Here's the drawing with two shaded views (mm, measured from the low corner). I have some questions. Round coordinates to 2 decimals unless told otherwise and drop trailing zeros. Write each loop counter-clockwise with the first axis right and the second up, starting at its lowest first coordinate (ties: lowest second). Pieces come first, ordered by that corner, then holes. Notation, with made-up numbers: M 62.25,89.25 L 68.25,89.25 A25 cw 68.25,127.25 Z; hole C 46,-38 d11. An arc over 180 degrees is marked long. Answer as a JSON object with one key per item and string values. Group by question number.
1) Suppose I cut it at B-B, the plane x = 28. Write out the boundary of the cut face in (y, z).
2) Suppose I cut it at C-C, the plane y = 21.5. Write out the boundary of the cut face in (x, z), and give its area (3 significant figures).
3) I'm going to push flat-ended pins straight in: pin 1 Ø1 at (y, z) = (2.5, 2.5) entering from -X; pin 2 Ø0.9 at (x, z) = (26.5, 1) entering from +Y. Where does each tip first touch, or does it pass through?
4) Please list where these lines run through material, in increasing order: L1, parallel to X at y = 23.75, z = 2.3; L2, parallel to X at y = 5, z = 1.1; L3, parallel to Y at x = 27, z = 1.6. Write a range as [from, to].
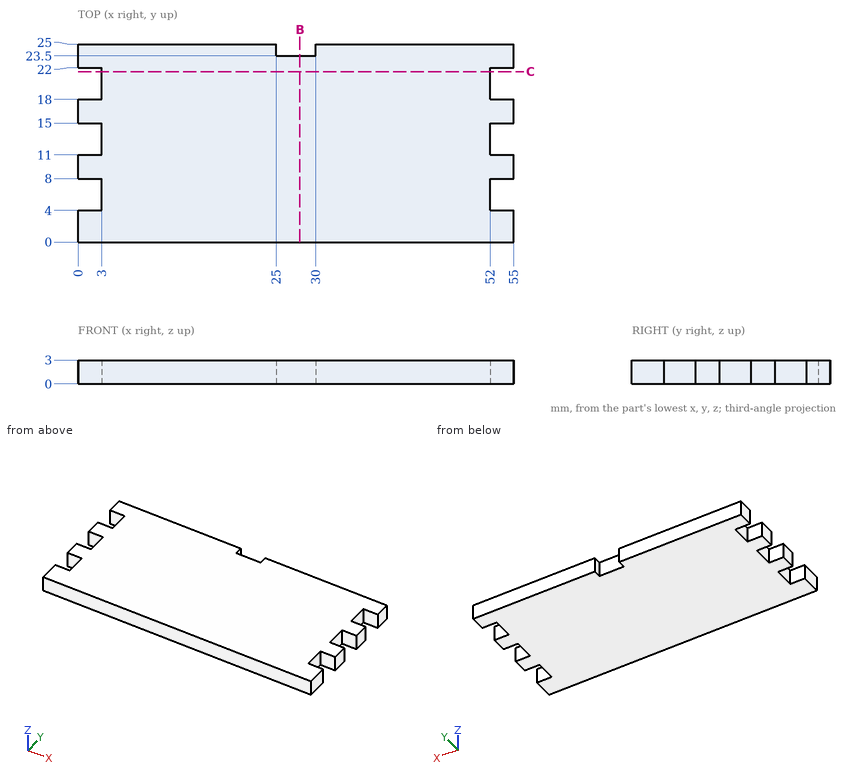
Results:
{
 "1": {"outline": "M 0,0 L 23.5,0 L 23.5,3 L 0,3 Z"},
 "2": {"outline": "M 3,0 L 52,0 L 52,3 L 3,3 Z", "area": "147 mm^2"},
 "3": {"pin 1": "x = 0", "pin 2": "y = 23.5"},
 "4": {"L1": "[0, 25], [30, 55]", "L2": "[3, 52]", "L3": "[0, 23.5]"}
}
